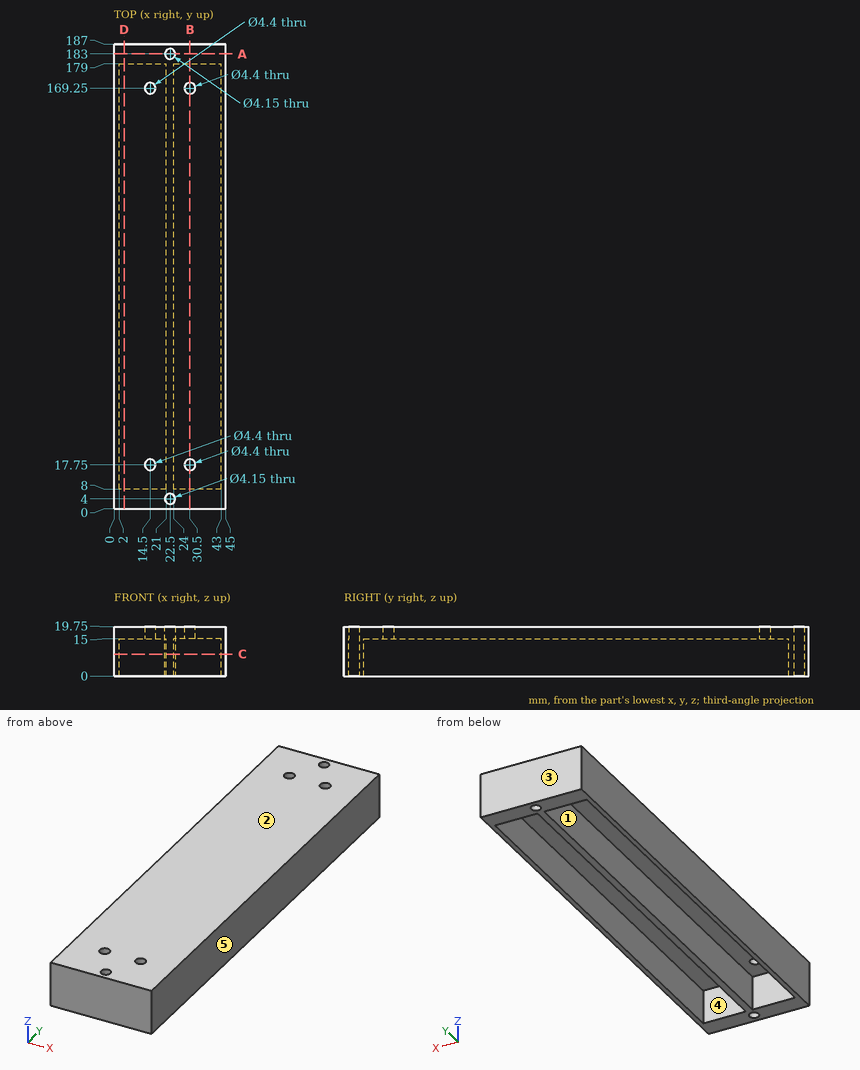
Geometry: see drawing. Coordinates: mm, zero at the bounding-box minimum. A direction names the side the tool comes from. Give positions to 0.01 mm unless a question says otherwise; leave off trailing zeros. Loops run counter-clockwise (first coordinate to the right, second up) from the corner with the lowest first, then second, coordinate; pieces in that order, holes last. Notation, with made-up numbers: (9.25, 46.5) - (34.25, 46.5) arc R12 ccw to (34.25, 61.5) - close; hole circle Ø8 at (-39, 21). An arc over 180 degrees is marked (long way). Use CSV: the item, a comma, the result in double quotes. Start each with the question number.
Item 1: Reachability of the marked faces 1 and 2 from +Z, -Z, +X, -X, +Y, -Y: full face, straight path, thin tool, end or side. Return the list, or none.
Item 2: Contact query for flat-ended pins moving along their axis: P1, Ø3.5, axis at x = 22.5, y = 183, coming from the -Z side; P2, Ø7.5, axis at y = 68, z = 9, coming from the -X side; P3, Ø5.5, axis at x = 12.5, y = 76.5, coming from the -Z side. Output: stop coordinate, or through.
Item 3: Section D-D on x = 4. Return loops of the section in (y, z).
Item 4: Mould query, pull axis X, two halves, no side actions, for the marked faces 3, 4 and 5. Classes: pulls with the +X half, pulls with the -X half, needs draft (parallel to the pull), parting line crosses it, or undercut.
Item 5: Line query: line 1 (X direction, y = 113.5, z = 6.25); line 2 (Y direction, x = 22.5, z = 5) (3 decimals); line 3 (Y direction, x = 14.5, z = 17.55). Output: solid intervals per line, ascending.
Item 6: Section A-A on y = 183. Return loops of the section in (x, z) (3 decimals), then the cut area to 3 significant figures.
Item 7: Section C-C on z = 8.75. Return loops of the section in (x, y) (3 decimals), then the cut area to 3 significant figures.
Item 8: Section B-B on x = 30.5. Return loops of the section in (y, z).
Ans:
1,face 1,"-Z"
1,face 2,"+Z, +X, -X, +Y, -Y"
2,P1,"passes through"
2,P2,"stops at x = 0"
2,P3,"stops at z = 15"
3,outline,"(0, 0) - (8, 0) - (8, 15) - (179, 15) - (179, 0) - (187, 0) - (187, 19.75) - (0, 19.75) - close"
4,face 3,"needs draft"
4,face 4,"undercut"
4,face 5,"pulls with the +X half"
5,line 1,"x = 0 to 2, 21 to 24, 43 to 45"
5,line 2,"y = 0 to 1.925, 6.075 to 180.925, 185.075 to 187"
5,line 3,"y = 0 to 15.55, 19.95 to 167.05, 171.45 to 187"
6,outline,"(0, 0) - (20.425, 0) - (20.425, 19.75) - (0, 19.75) - close; (24.575, 0) - (45, 0) - (45, 19.75) - (24.575, 19.75) - close"
6,area,"807 mm2"
7,outline,"(0, 0) - (45, 0) - (45, 187) - (0, 187) - close; hole (2, 8) - (21, 8) - (21, 179) - (2, 179) - close; hole circle Ø4.15 at (22.5, 4); hole circle Ø4.15 at (22.5, 183); hole (24, 8) - (43, 8) - (43, 179) - (24, 179) - close"
7,area,"1,890 mm2"
8,outline,"(0, 0) - (8, 0) - (8, 15) - (15.55, 15) - (15.55, 19.75) - (0, 19.75) - close; (19.95, 15) - (167.05, 15) - (167.05, 19.75) - (19.95, 19.75) - close; (171.45, 15) - (179, 15) - (179, 0) - (187, 0) - (187, 19.75) - (171.45, 19.75) - close"
